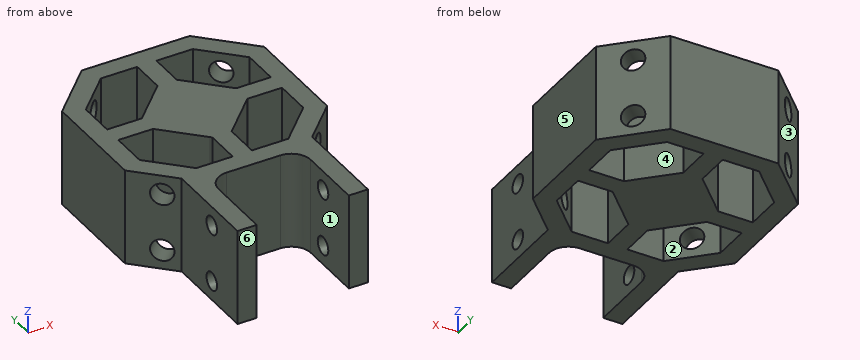
```python
from build123d import *

# Parameters (mm, degrees)
EXTRUDE_THIN1_DEPTH = 25
SKETCH5_W           = 23.970919882
SKETCH5_H           = 5
BOSS_EXTRUDE2_DEPTH = 25
BOSS_EXTRUDE3_DEPTH = 25
SKETCH6_R           = 2.85
CUT_EXTRUDE1_DEPTH  = 5
SKETCH9_R           = 2.85
CUT_EXTRUDE2_DEPTH  = 5
CUT_EXTRUDE3_START  = -5
SKETCH10_R          = 2.85
CUT_EXTRUDE3_DEPTH  = 5
CUT_EXTRUDE4_START  = -5
SKETCH11_R          = 2.85
CUT_EXTRUDE4_DEPTH  = 5
FILLET1_R           = 5
CUT_EXTRUDE5_REACH  = 91.834
SKETCH12_R          = 2.35


with BuildPart() as part:
    # Sketch1 → Extrude-Thin1 (new body)
    with BuildSketch(Plane.XY):
        Polygon((11.985459941, 0), (11.985459941, 26.992888143), (21.319269453, 36.326697654), (21.319269453, 60.297617537), (11.985459941, 69.631427048), (-11.985459941, 69.631427048), (-21.319269453, 60.297617537), (-21.319269453, 36.326697654), (-11.985459941, 26.992888143), (-11.985459941, 0), (-16.985459941, 0), (-16.985459941, 24.921820331), (-26.319269453, 34.255629842), (-26.319269453, 62.368685348), (-14.056527753, 74.631427048), (14.056527753, 74.631427048), (26.319269453, 62.368685348), (26.319269453, 34.255629842), (16.985459941, 24.921820331), (16.985459941, 0), align=None)
    extrude(amount=-EXTRUDE_THIN1_DEPTH)

    # Sketch5 → Boss-Extrude2 (add)
    with BuildSketch(Plane.XY):
        with Locations((0, 24.492888143)):
            Rectangle(SKETCH5_W, SKETCH5_H)
    extrude(amount=-BOSS_EXTRUDE2_DEPTH)

    # Sketch3 → Boss-Extrude3 (add)
    with BuildSketch(Plane.XY):
        Polygon((-2.5, 36.033625869), (-2.5, 26.992888143), (2.5, 26.992888143), (2.5, 36.033625869), (2.899137803, 36.432763672), (11.879393924, 45.413019793), (12.278531727, 45.812157595), (21.319269453, 45.812157595), (21.319269453, 50.812157595), (12.278531727, 50.812157595), (11.879393924, 51.211295398), (2.899137803, 60.191551519), (2.5, 60.590689322), (2.5, 69.631427048), (-2.5, 69.631427048), (-2.5, 60.590689322), (-2.899137803, 60.191551519), (-12.278531727, 50.812157595), (-21.319269453, 50.812157595), (-21.319269453, 45.812157595), (-12.278531727, 45.812157595), (-2.899137803, 36.432763672), align=None)
    extrude(amount=-BOSS_EXTRUDE3_DEPTH)

    # Sketch6 → Cut-Extrude1 (cut)
    with BuildSketch(Plane(origin=(3.968180195, 3.968180195, 0), x_dir=(0, 0, 1), z_dir=(-0.7071067811865479, -0.7071067811865471, 0))):
        with Locations(Location((-20, 34.161854249, 0), (0, 0, 270))):
            Circle(SKETCH6_R)
        with Locations(Location((-5, 34.161854249, 0), (0, 0, 270))):
            Circle(SKETCH6_R)
    extrude(amount=-CUT_EXTRUDE1_DEPTH, mode=Mode.SUBTRACT)

    # Sketch9 → Cut-Extrude2 (cut)
    with BuildSketch(Plane(origin=(-3.968180195, 3.968180195, 0), x_dir=(0, 0, 1), z_dir=(0.7071067811865479, -0.7071067811865471, 0))):
        with Locations(Location((-20, -34.161854249, 0), (0, 0, 270))):
            Circle(SKETCH9_R)
        with Locations(Location((-5, -34.161854249, 0), (0, 0, 270))):
            Circle(SKETCH9_R)
    extrude(amount=-CUT_EXTRUDE2_DEPTH, mode=Mode.SUBTRACT)

    # Sketch10 → Cut-Extrude3 (cut)
    with BuildSketch(Plane(origin=(-44.343977401, 44.343977401, 0), x_dir=(0, 0, 1), z_dir=(-0.7071067811865471, 0.707106781186548, 0)).offset(CUT_EXTRUDE3_START)):
        with Locations(Location((-20, 34.161854249, 0), (0, 0, 90))):
            Circle(SKETCH10_R)
        with Locations(Location((-5, 34.161854249, 0), (0, 0, 90))):
            Circle(SKETCH10_R)
    extrude(amount=CUT_EXTRUDE3_DEPTH, mode=Mode.SUBTRACT)

    # Sketch11 → Cut-Extrude4 (cut)
    with BuildSketch(Plane(origin=(44.343977401, 44.343977401, 0), x_dir=(0, 0, -1), z_dir=(0.7071067811865471, 0.707106781186548, 0)).offset(CUT_EXTRUDE4_START)):
        with Locations(Location((5, 34.161854249, 0), (0, 0, 270))):
            Circle(SKETCH11_R)
        with Locations(Location((20, 34.161854249, 0), (0, 0, 270))):
            Circle(SKETCH11_R)
    extrude(amount=CUT_EXTRUDE4_DEPTH, mode=Mode.SUBTRACT)

    # Fillet1
    fillet1_edges = [part.edges().sort_by_distance(p)[0] for p in [
        (11.985459941, 21.992888143, -12.5),
        (-11.985459941, 21.992888143, -12.5),
    ]]
    fillet(fillet1_edges, radius=FILLET1_R)

    # Cut-Extrude5: up to this face of the body (flat: up to its plane)
    cut_extrude5_end = Plane(part.part.faces().sort_by_distance((-16.985459941, 12.460910165, -12.5))[0])
    # Sketch12 → Cut-Extrude5 (cut, up to the picked face)
    with BuildSketch(Plane(origin=(16.985459941, 0, 0), x_dir=(0, 0, -1), z_dir=(1, 0, 0)), mode=Mode.PRIVATE) as cut_extrude5_sk1:
        with Locations(Location((20, 11.5, 0), (0, 0, 90))):
            Circle(SKETCH12_R)
    cut_extrude5_tool1 = split(extrude(cut_extrude5_sk1.sketch, amount=-CUT_EXTRUDE5_REACH, mode=Mode.PRIVATE), bisect_by=cut_extrude5_end, keep=Keep.BOTH, mode=Mode.PRIVATE)
    # Sketch12 → Cut-Extrude5 (cut, up to the picked face)
    with BuildSketch(Plane(origin=(16.985459941, 0, 0), x_dir=(0, 0, -1), z_dir=(1, 0, 0)), mode=Mode.PRIVATE) as cut_extrude5_sk2:
        with Locations(Location((5, 11.5, 0), (0, 0, 90))):
            Circle(SKETCH12_R)
    cut_extrude5_tool2 = split(extrude(cut_extrude5_sk2.sketch, amount=-CUT_EXTRUDE5_REACH, mode=Mode.PRIVATE), bisect_by=cut_extrude5_end, keep=Keep.BOTH, mode=Mode.PRIVATE)
    add(cut_extrude5_tool1.solids().sort_by(Axis((16.98546, 11.5, -20), (-1, 0, 0)))[0], mode=Mode.SUBTRACT)
    add(cut_extrude5_tool2.solids().sort_by(Axis((16.98546, 11.5, -5), (-1, 0, 0)))[0], mode=Mode.SUBTRACT)


solid = part.part
```
Part model, mm, in its own coordinate system. Face numbers are marked on the shaded views. A direction names the side the tool comes from. Round coordinates to 2 decimals unless told otherwise and drop trailing zeros. Order: outer loops, then holes, each group sorted by start corner. A loop starts at its lowest first (then second) coordinate and runs counter-clockwise, first axis right, second up. Notation, with made-up numbers: M 45.25,29.5 L 72.25,29.5 A23 cw 72.25,50.5 Z; hole C 66,19 d7. An arc over 180 degrees is marked long. Put each result on its own line as item: value. Start each with the question number.
1. Slice it at A-A on x = 9.5. List the corners of the cut face in (y, z).
2. Drop flat-ended pins along their axis: pin 1 (3 mm diameter, centred on x = -1, y = 20, fed in from -Z); pin 2 (2 mm diameter, centred on y = 17.5, z = -20, fed in from -X); pin 3 (6 mm diameter, centred on y = 11.5, z = -5, fed in from +X); pin 4 (7 mm diameter, centred on y = 29.5, z = -18, fed in from +X). Give the stop position or say it passes through.
3. Slice it at D-D on z = -10.5. State how many separate pieces and enclosed holes the cut face has, then the cut area to 3 significant figures.
4. Drill centre lines: probe 1 along Z at (x, y) = (14.95, 11.5); probe 2 along X at (y, z) = (5.5, -22.5); probe 3 along Y at (x, z) = (3, -3.75). Where is each one in solid material? Low to high. Write a range as [from, to].
5. Slice it at C-C on y = 44. List the corners of the cut face in (x, z), then the cut area to 3 significant figures.
6. Two-plate mould, pull along X, no slides. Class the marked faces 4, 5 and 6: +X half, -X half, draft (parallel to the pull), parting line (faces both ways), or undercut.
7. Slice it at B-B on y = 11.5. List the corners of the cut face in (x, z), then the cut area to 3 significant figures.
8. Tool access for the marked faces 1, 2 and 3: list every direction of +Z, -Z, +X, -X, +Y, -Y with a clear straight run to the whole face (end or side of a thin tool).
Findings:
1. outline: M 21.31,-25 L 26.99,-25 L 26.99,0 L 21.31,0 Z; M 43.03,-25 L 53.59,-25 L 53.59,0 L 43.03,0 Z; M 69.63,-25 L 74.63,-25 L 74.63,0 L 69.63,0 Z
2. pin 1: through
2. pin 2: x = -16.99
2. pin 3: x = 16.99
2. pin 4: x = 25.06
3. separate pieces: 1
3. enclosed holes: 4
3. area: 1,660 mm2
4. probe 1: [-25, -22.35], [-17.65, -7.35], [-2.65, 0]
4. probe 2: [-16.99, -11.99], [11.99, 16.99]
4. probe 3: [21.99, 26.99], [36.53, 60.09], [69.63, 74.63]
5. outline: M -26.32,-25 L -21.32,-25 L -21.32,0 L -26.32,0 Z; M -10.47,-25 L 10.47,-25 L 10.47,0 L -10.47,0 Z; M 21.32,-25 L 26.32,-25 L 26.32,0 L 21.32,0 Z
5. area: 773 mm2
6. face 4: undercut
6. face 5: +X half
6. face 6: draft
7. outline: M -16.99,-25 L -11.99,-25 L -11.99,-22.35 L -16.99,-22.35 Z; M -16.99,-17.65 L -11.99,-17.65 L -11.99,-7.35 L -16.99,-7.35 Z; M -16.99,-2.65 L -11.99,-2.65 L -11.99,0 L -16.99,0 Z; M 11.99,-25 L 16.99,-25 L 16.99,-22.35 L 11.99,-22.35 Z; M 11.99,-17.65 L 16.99,-17.65 L 16.99,-7.35 L 11.99,-7.35 Z; M 11.99,-2.65 L 16.99,-2.65 L 16.99,0 L 11.99,0 Z
7. area: 156 mm2
8. face 1: +Z, -Z, -Y
8. face 2: +Z, -Z
8. face 3: +Z, -Z, -X, +Y
